Work out the finished part from the listing and answer in its coordinate system (mm). A direction names the side the tool comes from. Round coordinates to 2 decimals unless told otherwise and drop trailing zeros. Write each loop counter-clockwise with the first axis right and the second up, starting at its lowest first coordinate (ties: lowest second). Pieces come first, ordered by that corner, then holes. Notation, with made-up numbers: (26, 65) - (84, 65) arc R16 ccw to (84, 77) - close; hole circle Ø8 at (-2, -21.75). An arc over 180 degrees is marked (long way). Answer as a JSON object with one key per item and string values.
```python
from build123d import *

# Parameters (mm, degrees)
SKETCH1_W                  = 40
SKETCH1_H                  = 20
BOSS_EXTRUDE1_DEPTH        = 40
SKETCH2_W                  = 20
SKETCH2_H                  = 3
BOSS_EXTRUDE2_DEPTH        = 7.4
SKETCH3_R                  = 2.9
BOSS_EXTRUDE3_DEPTH        = 5.8
SKETCH5_R                  = 6.5
BOSS_EXTRUDE4_DEPTH        = 1.6
M2_5_CLEARANCE_SLOT1_D     = 2.9
M2_5_CLEARANCE_SLOT1_DEPTH = 8.999
M2_5_CLEARANCE_SLOT1_TIP   = 0.871247898


with BuildPart() as part:
    # Sketch1 → Boss-Extrude1 (new body)
    with BuildSketch(Plane(origin=(0, 0, 0), x_dir=(1, 0, 0), z_dir=(0, 1, 0))):
        Rectangle(SKETCH1_W, SKETCH1_H)
    extrude(amount=BOSS_EXTRUDE1_DEPTH)

    # Sketch2 → Boss-Extrude2 (add)
    with BuildSketch(Plane(origin=(20, 0, 0), x_dir=(0, 0, -1), z_dir=(1, 0, 0))):
        with Locations((0, 29)):
            Rectangle(SKETCH2_W, SKETCH2_H)
    boss_extrude2 = extrude(amount=BOSS_EXTRUDE2_DEPTH)

    # Mirror1: Boss-Extrude2 across plane
    add(boss_extrude2.mirror(Plane(origin=(0, 0, 0), x_dir=(0, 0, 1), z_dir=(1, 0, 0))))

    # Sketch3 → Boss-Extrude3 (add)
    with BuildSketch(Plane(origin=(0, 40, 0), x_dir=(1, 0, 0), z_dir=(0, 1, 0))):
        with Locations((10.5, 0)):
            Circle(SKETCH3_R)
    extrude(amount=BOSS_EXTRUDE3_DEPTH)

    # Sketch5 → Boss-Extrude4 (add)
    with BuildSketch(Plane(origin=(0, 40, 0), x_dir=(1, 0, 0), z_dir=(0, 1, 0))):
        with Locations((10.5, 0)):
            Circle(SKETCH5_R)
    extrude(amount=BOSS_EXTRUDE4_DEPTH)

    # M2.5 Clearance Slot1
    with Locations(Plane(origin=(-162.114339431, 30.5, -5.431907662), x_dir=(0.412719532, 0, 0.91085816), z_dir=(0, 1, 0))):
        with Locations((57.189532403, 125.168887287), (66.298114004, 121.041691966), (77.412789478, 169.800937131), (86.521371079, 165.67374181)):
            Hole(M2_5_CLEARANCE_SLOT1_D / 2, depth=M2_5_CLEARANCE_SLOT1_DEPTH)
            with Locations((0, 0, -(M2_5_CLEARANCE_SLOT1_DEPTH + M2_5_CLEARANCE_SLOT1_TIP / 2))):  # 118° drill point
                Cone(0, M2_5_CLEARANCE_SLOT1_D / 2, M2_5_CLEARANCE_SLOT1_TIP, mode=Mode.SUBTRACT)


solid = part.part
```
Item 1: Each of these flat-tipped pins is pushed along its axis until it touches: P1, Ø8, axis at y = 8.5, z = 1.5, coming from the -X side; P2, Ø6, axis at y = 16, z = 4, coming from the +X side; P3, Ø8, axis at x = 25, z = 0, coming from the +Y side; P4, Ø8, axis at x = -9, z = -1.5, coming from the -Y side. Where does it stop, or does it pass through?
Results found:
{"P1": "x = -20", "P2": "x = 20", "P3": "y = 30.5", "P4": "y = 0"}
Item 2: A cutting plane is placed at A-A (x = -24.5). Write down the section's boundary in (y, z).
Results found:
{"outline": "(27.5, -10) - (30.5, -10) - (30.5, -6.45) - (27.5, -6.45) - close; (27.5, -3.55) - (30.5, -3.55) - (30.5, 3.55) - (27.5, 3.55) - close; (27.5, 6.45) - (30.5, 6.45) - (30.5, 10) - (27.5, 10) - close"}
Item 3: A cutting plane is placed at B-B (z = -5). Write down the section's boundary in (x, y), and give its area (3 significant figures).
Results found:
{"outline": "(-27.4, 27.5) - (-25.95, 27.5) - (-25.95, 30.5) - (-27.4, 30.5) - close; (-23.05, 27.5) - (-20, 27.5) - (-20, 0) - (20, 0) - (20, 27.5) - (23.05, 27.5) - (23.05, 30.5) - (20, 30.5) - (20, 40) - (14.65, 40) - (14.65, 41.6) - (6.35, 41.6) - (6.35, 40) - (-20, 40) - (-20, 30.5) - (-23.05, 30.5) - close; (25.95, 27.5) - (27.4, 27.5) - (27.4, 30.5) - (25.95, 30.5) - close", "area": "1,640 mm²"}
Item 4: Determine the mould class of faces 1 (the cylindrical face through (25.834, 28.979, -4.431)), 2 (the cylindrical face through (7.6, 43.7, -0.1)), 3 (the flat face through (24, 27.5, 0)) for opening direction X: pulls with the +X half, pulls with the -X half, needs draft (parallel to the pull), parting line crosses it, or undercut.
Results found:
{"face 1": "undercut", "face 2": "parting line crosses it", "face 3": "needs draft"}
Item 5: Consider line 1 along X through (y, z) = (28.8, 5); line 2 along Z through (x, y) = (-24.5, 28.8); line 3 along Y through (x, z) = (4.5, -6.5). Determine where each line is inside the solid, lowest interval first.
Results found:
{"line 1": "-27.4 to -25.95, -23.05 to 23.05, 25.95 to 27.4", "line 2": "-10 to -6.45, -3.55 to 3.55, 6.45 to 10", "line 3": "0 to 40"}
Item 6: For faces 4 (the flat face through (13.3, 41.6, 1.4)), 5 (the flat face through (-24, 27.5, 0)), 6 (the flat face through (-24, 30.5, 0)), determine the directions among +Z, -Z, +X, -X, +Y, -Y from which every point of the face is accessible in a straight line to the end or side of a thin tool.
Results found:
{"face 4": "+Y", "face 5": "+Z, -Z, -X, -Y", "face 6": "+Z, -Z, -X, +Y"}
Item 7: A cutting plane is placed at D-D (y = 7.5). Write down the section's boundary in (x, z).
Results found:
{"outline": "(-20, -10) - (20, -10) - (20, 10) - (-20, 10) - close"}
Item 8: A cutting plane is placed at C-C (x = 10.5). Write down the section's boundary in (y, z).
Results found:
{"outline": "(0, -10) - (40, -10) - (40, -6.5) - (41.6, -6.5) - (41.6, -2.9) - (45.8, -2.9) - (45.8, 2.9) - (41.6, 2.9) - (41.6, 6.5) - (40, 6.5) - (40, 10) - (0, 10) - close"}
